```python
from build123d import *

# Parameters (mm, degrees)
FOOTPRINT_DEPTH = 1
CHAMFER1_SIZE   = 0.5


with BuildPart() as part:
    # Sketch1 → Body (revolve)
    with BuildSketch(Plane(origin=(0, 0, 0), x_dir=(0, 0, -1), z_dir=(1, 0, 0)), mode=Mode.PRIVATE) as body_sk:
        Polygon((0, 0), (0, 2), (2, 1), (12, 1), (12, 0), align=None)
    revolve(body_sk.sketch.rotate(Axis((0, 0, 58.51474448), (0, 0, -1)), 90), axis=Axis((0, 0, 58.51474448), (0, 0, -1)))

    # Sketch2 → Footprint (cut)
    with BuildSketch(Plane.XY):
        Polygon((0, 1.154700538), (-1, 0.577350269), (-1, -0.577350269), (0, -1.154700538), (1, -0.577350269), (1, 0.577350269), align=None)
    extrude(amount=-FOOTPRINT_DEPTH, mode=Mode.SUBTRACT)

    # Chamfer1
    chamfer1_edges = [part.edges().sort_by_distance(p)[0] for p in [
        (-1, 0, -12),
    ]]
    chamfer(chamfer1_edges, length=CHAMFER1_SIZE)


solid = part.part
```
Could you check a few things on this model? Use its own coordinates, in mm. A direction names the side the tool comes from. Give positions to 0.01 mm unless a question says otherwise; leave off trailing zeros. Loops run counter-clockwise (first coordinate to the right, second up) from the corner with the lowest first, then second, coordinate; pieces in that order, holes last. Notation, with made-up numbers: (-11, -6.5) - (15, -6.5) arc R34 ccw to (15, 23.5) - close; hole circle Ø8 at (72, 1.25). An arc over 180 degrees is marked (long way). Answer in a Markdown table with one row per item. Add a question column.
Q1. If we section it at A-A (y = 0): List the corners of the cut face in (x, z) for me, plus the area to 4 significant figures.
Q2. We'd pull the mould along Y, two halves only. Please class faces 1 (the face through (-0.15, -1.15, -1.68)), 2 (the face through (0, 0, -12)), 3 (the face through (0.49, -0.87, -0.49)): +Y half, -Y half, draft (parallel to the pull), parting line (faces both ways), or undercut.
Q3. If we section it at C-C (z = -1.75): List the corners of the cut face in (x, y) for me (3 decimals), plus the area to 3 significant figures.
Q4. If we section it at B-B (z = -7): List the corners of the cut face in (x, y) for me, plus the area to 3 significant figures.
Q5. For pin 1 (2 mm diameter, centred on x = -0.5, z = -7.5, fed in from -Y); pin 2 (1.1 mm diameter, centred on y = 0, z = -0.5, fed in from -X); pin 3 (0.5 mm diameter, centred on y = 0, z = -0.5, fed in from +X) (3 decimals), each with a flat end and sliding along its axis, tell me the tip position at first contact or that it passes through.
Q6. Which directions (+Z, -Z, +X, -X, +Y, -Y) give clear straight access to the entire face, cutting with the end or side of a thin tool? Please do faces 4 (the face through (0, 1, -7)), 5 (the face through (-1, 1, 0)), 6 (the face through (-0.49, 0.87, -0.49)).
Q7. Please list where these lines run through material, in increasing order: L1, parallel to X at y = 0.4, z = -0.75 (3 decimals); L2, parallel to Y at x = -0.05, z = -6; L3, parallel to Z at x = -0.4, y = -0.15. Write a range as from..to.
The answers:
| question | item | result |
|---|---|---|
| 1 | outline | (-2, 0) - (-1, -2) - (-1, -11.5) - (-0.5, -12) - (0.5, -12) - (1, -11.5) - (1, -2) - (2, 0) - (1, 0) - (1, -1) - (-1, -1) - (-1, 0) - close |
| 1 | area | 23.75 mm^2 |
| 2 | face 1 | parting line |
| 2 | face 2 | draft |
| 2 | face 3 | undercut |
| 3 | outline | circle Ø2.25 at (0, 0) |
| 3 | area | 3.98 mm^2 |
| 4 | outline | circle Ø2 at (0, 0) |
| 4 | area | 3.14 mm^2 |
| 5 | pin 1 | stops at y = -1 |
| 5 | pin 2 | stops at x = -2 |
| 5 | pin 3 | stops at x = 1.875 |
| 6 | face 4 | -Z |
| 6 | face 5 | +Z, +X, -X, +Y, -Y |
| 6 | face 6 | +Z |
| 7 | L1 | x = -1.575..-1, 1..1.575 |
| 7 | L2 | y = -1..1 |
| 7 | L3 | z = -12..-1 |
